Could you check a few things on this model? Use its own coordinates, in mm. A direction names the side the tool comes from. Give positions to 0.01 mm unless a question says otherwise; leave off trailing zeros. Order: outer loops, then holes, each group sorted by start corner. A loop starts at its lowest first (then second) coordinate and runs counter-clockwise, first axis right, second up.
from build123d import *

# Parameters (mm, degrees)
F0_W     = 90
F0_H     = 18
F0_R     = 2.25
F1_DEPTH = 3
F2_W     = 8
F2_H     = 18
F3_DEPTH = 15
F4_R     = 2.4
F5_DEPTH = 18


with BuildPart() as f1:
    # F0 (on Top) → F1 (new body)
    with BuildSketch(Plane.XY):
        with Locations((3.318636, 0)):
            Rectangle(F0_W, F0_H)
        with Locations((-34.681364, 0)):
            Circle(F0_R, mode=Mode.SUBTRACT)
        with Locations((28.318636, 0)):
            Circle(F0_R, mode=Mode.SUBTRACT)
    extrude(amount=F1_DEPTH)

    # F2 (on face) → F3 (join)
    with BuildSketch(Plane.XY.offset(3)):
        with Locations((37.318636, 0)):
            Rectangle(F2_W, F2_H)
    extrude(amount=F3_DEPTH)

    # F4 (on face) → F5 (cut, through all)
    with BuildSketch(Plane(origin=(0, 9, 0), x_dir=(-1, 0, 0), z_dir=(0, 1, 0))):
        with Locations((-37.318636, 13)):
            Circle(F4_R)
    extrude(amount=-F5_DEPTH, mode=Mode.SUBTRACT)


solid = f1.part
Item 1: Imagine slicing it at C-C on y = -7. List the corners of the cut face in (x, z) for me, then the cut area to 3 significant figures.
Findings:
outline: (-41.68, 0) - (48.32, 0) - (48.32, 3) - (41.32, 3) - (41.32, 18) - (33.32, 18) - (33.32, 3) - (-41.68, 3) - close; hole circle Ø4.8 at (37.32, 13)
area: 372 mm2
Item 2: For pin 1 (1 mm diameter, centred on y = -4, z = 9.5, fed in from -X); pin 2 (7.5 mm diameter, centred on x = 46, y = 3, fed in from +Z); pin 3 (8 mm diameter, centred on y = 3, z = 5.5, fed in from -X), each with a flat end and sliding along its axis, tell me the tip position at first contact or that it passes through.
Findings:
pin 1: stops at x = 33.32
pin 2: stops at z = 3
pin 3: stops at x = -41.68
Item 3: For faces 1 (the flat face through (45, 0, 3)), 2 (the flat face through (33.319, 0, 10)), 3 (the flat face through (48.319, 0, 1)), which set-ups out of +Z, -Z, +X, -X, +Y, -Y let a thin tool reach every point of the face, with its end or its side?
Findings:
face 1: +Z, +X, +Y, -Y
face 2: +Z, -X, +Y, -Y
face 3: +Z, -Z, +X, +Y, -Y
Item 4: Imagine slicing it at D-D on x = 29.5. List the corners of the cut face in (y, z) for me.
Findings:
outline: (-9, 0) - (-1.91, 0) - (-1.91, 3) - (-9, 3) - close; (1.91, 0) - (9, 0) - (9, 3) - (1.91, 3) - close
Item 5: Please list where these lines run through material, in increasing order: line 1 along Z through (x, y) = (37.5, -5.75); line 2 along Z through (x, y) = (22.5, 4.25); line 3 along X through (y, z) = (-5, 7.25).
Findings:
line 1: z = 0 to 10.61, 15.39 to 18
line 2: z = 0 to 3
line 3: x = 33.32 to 41.32
Item 6: Imagine slicing it at B-B on z = 13. List the corners of the cut face in (x, y) for me.
Findings:
outline: (33.32, -9) - (34.92, -9) - (34.92, 9) - (33.32, 9) - close; (39.72, -9) - (41.32, -9) - (41.32, 9) - (39.72, 9) - close
Item 7: Imagine slicing it at A-A on y = 0. List the corners of the cut face in (x, z) for me.
Findings:
outline: (-41.68, 0) - (-36.93, 0) - (-36.93, 3) - (-41.68, 3) - close; (-32.43, 0) - (26.07, 0) - (26.07, 3) - (-32.43, 3) - close; (30.57, 0) - (48.32, 0) - (48.32, 3) - (41.32, 3) - (41.32, 18) - (33.32, 18) - (33.32, 3) - (30.57, 3) - close; hole circle Ø4.8 at (37.32, 13)
Item 8: We'd pull the mould along Y, two halves only. Please class faces 4 (the flat face through (10, 9, 2)), 5 (the cylindrical face through (-36.93, 0.1, 1.48)), 6 (the flat face through (41.319, 0, 10)): +Y half, -Y half, draft (parallel to the pull), parting line (faces both ways), or undercut.
Findings:
face 4: +Y half
face 5: undercut
face 6: draft
